Could you check a few things on this drawing? It's one solid part, dimensions in mm from its lowest x, y, z. Give positions to 0.01 mm unless a question says otherwise; leave off trailing zeros. Order: outer loops, then holes, each group sorted by start corner. A loop starts at its lowest first (then second) coordinate and runs counter-clockwise, first axis right, second up. Notation, with made-up numbers: M 23.25,9.25 L 27.25,9.25 A20 ccw 27.25,38.25 Z; hole C -29,11 d11. An arc over 180 degrees is marked long. Use one line per item in the form item = value.
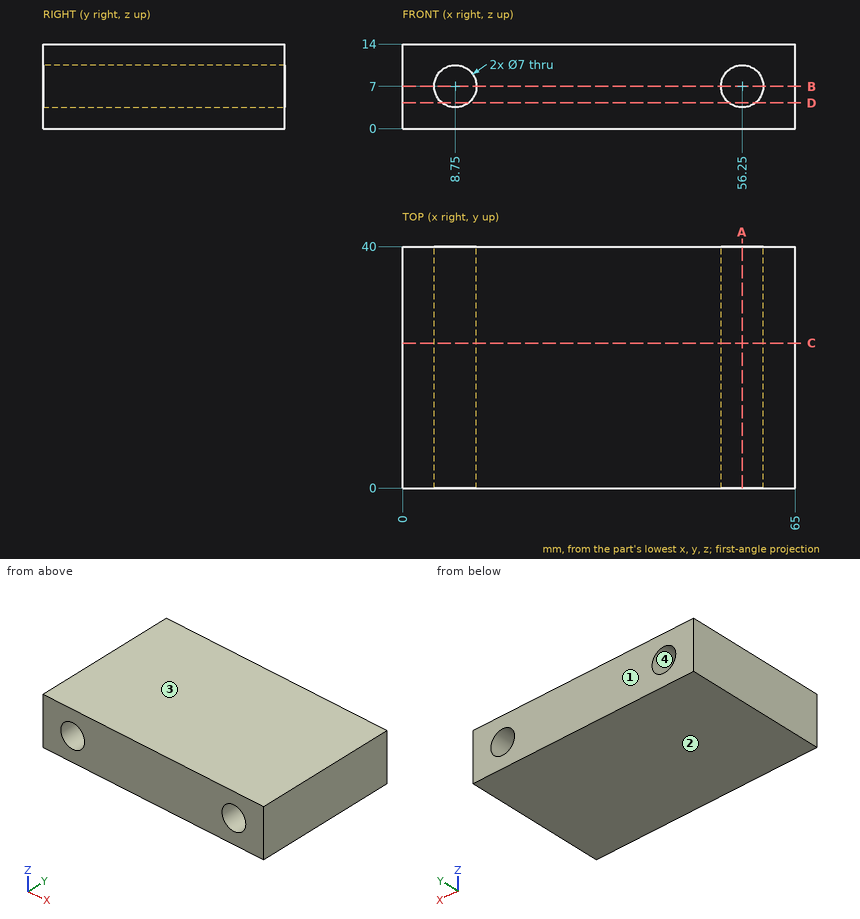
Q1. I want a section at B-B on z = 7. Write out the boundary of the cut face in (x, y), then the cut area to 3 significant figures.
Found:
outline = M 0,0 L 5.25,0 L 5.25,40 L 0,40 Z; M 12.25,0 L 52.75,0 L 52.75,40 L 12.25,40 Z; M 59.75,0 L 65,0 L 65,40 L 59.75,40 Z
area = 2,040 mm²
Q2. I want a section at D-D on z = 4.25. Write out the boundary of the cut face in (x, y).
Found:
outline = M 0,0 L 6.58,0 L 6.58,40 L 0,40 Z; M 10.92,0 L 54.08,0 L 54.08,40 L 10.92,40 Z; M 58.42,0 L 65,0 L 65,40 L 58.42,40 Z
Q3. I want a section at A-A on x = 56.25. Write out the boundary of the cut face in (y, z).
Found:
outline = M 0,0 L 40,0 L 40,3.5 L 0,3.5 Z; M 0,10.5 L 40,10.5 L 40,14 L 0,14 Z
Q4. Thinking about a two-plate mould opening in Z: for the marked faces 1, 2, 3 and 4, which applies, +Z half, -Z half, draft (parallel to the pull), parting line (faces both ways), or undercut?
Found:
face_1 = draft
face_2 = -Z half
face_3 = +Z half
face_4 = undercut
Q5. I'm going to push flat-ended pins straight in: pin 1 Ø1 at (x, y) = (50, 32) entering from -Z; pin 2 Ø4 at (x, z) = (8.75, 7) entering from +Y. Where does each tip first touch, or does it pass through?
Found:
pin_1 = 0
pin_2 = through
Q6. I want a section at C-C on y = 24. Write out the boundary of the cut face in (x, z), then the cut area to 3 significant figures.
Found:
outline = M 0,0 L 65,0 L 65,14 L 0,14 Z; hole C 8.75,7 d7; hole C 56.25,7 d7
area = 833 mm²
Q7. I need wall thicknesses on L1, parallel to X at y = 28.5, z = 7; L2, parallel to X at y = 11, z = 9.25; L3, parallel to Z at x = 56, y = 20. Which ranges of each line are inside material? Lowest first, please.
Found:
L1 = 0 to 5.25, 12.25 to 52.75, 59.75 to 65
L2 = 0 to 6.07, 11.43 to 53.57, 58.93 to 65
L3 = 0 to 3.51, 10.49 to 14
